CAD build for the part. Positions are in the model's coordinates, mm. A direction names the side the tool comes from. Round coordinates to 2 decimals unless told otherwise and drop trailing zeros. Loops run counter-clockwise (first coordinate to the right, second up) from the corner with the lowest first, then second, coordinate; pieces in that order, holes last. Notation, with made-up numbers: M 6,52 L 48,52 A18 cw 48,58 Z; hole C 22,-5 d1. An arc over 180 degrees is marked long. Put each result on its own line as item: value. Start each with the question number.
from build123d import *

# Parameters (mm, degrees)
PAD_DEPTH       = 5
FILLET_R        = 1
FILLET001_R     = 1
FILLET002_R     = 1
SKETCH001_R     = 1.75
PAD001_DEPTH    = 2
SKETCH002_W     = 61.2
SKETCH002_H     = 76.2
PAD002_DEPTH    = 2
PAD003_DEPTH    = 55
SKETCH004_W     = 35
SKETCH004_H     = 25
SKETCH004_W_2   = 14.2
SKETCH004_H_2   = 19
SKETCH004_W_3   = 51.2
SKETCH004_H_3   = 20
POCKET_DEPTH    = 2
SKETCH005_W     = 14.2
SKETCH005_H     = 19
SKETCH005_W_2   = 51.2
SKETCH005_H_2   = 20
POCKET001_DEPTH = 2
SKETCH006_W     = 66.2
SKETCH006_H     = 22
SKETCH006_H_2   = 17
POCKET002_DEPTH = 2
SKETCH007_W     = 24.2
SKETCH007_H     = 10
SKETCH007_W_2   = 31.5
SKETCH007_H_2   = 12
SKETCH007_R     = 1.25
PAD004_DEPTH    = 2
SKETCH008_W     = 31.5
SKETCH008_H     = 2
PAD005_DEPTH    = 3
PAD006_DEPTH    = 2
SKETCH010_W     = 5
SKETCH010_H     = 3
PAD007_DEPTH    = 2
SKETCH011_W     = 6
SKETCH011_H     = 6
SKETCH011_R     = 1.25
PAD008_DEPTH    = 6
SKETCH012_W     = 2
SKETCH012_H     = 10
PAD009_DEPTH    = 25


with BuildPart() as part:
    # Sketch → Pad (new body)
    with BuildSketch(Plane.XY):
        Polygon((28.537386, 0), (-14.268693, 24.714102), (-14.268693, -24.714102), align=None)
        Polygon((24.537386, 0), (-12.268693, 21.25), (-12.268693, -21.25), align=None, mode=Mode.SUBTRACT)
    extrude(amount=PAD_DEPTH)

    # Fillet
    fillet_edges = [part.edges().sort_by_distance(p)[0] for p in [
        (-14.268693, -24.714102, 2.5),
    ]]
    fillet(fillet_edges, radius=FILLET_R)

    # Fillet001
    fillet001_edges = [part.edges().sort_by_distance(p)[0] for p in [
        (28.537386, 0, 2.5),
    ]]
    fillet(fillet001_edges, radius=FILLET001_R)

    # Fillet002
    fillet002_edges = [part.edges().sort_by_distance(p)[0] for p in [
        (-14.268693, 24.714102, 2.5),
    ]]
    fillet(fillet002_edges, radius=FILLET002_R)

    # Sketch001 (on Face1 of Fillet002) → Pad001 (join)
    with BuildSketch(Plane(origin=(0, 0, 0), x_dir=(1, 0, 0), z_dir=(0, 0, -1))):
        Polygon((24.537386, 0), (-12.268693, 21.25), (-12.268693, -21.25), align=None)
        with Locations((4.134347, 7.160898)):
            Circle(SKETCH001_R, mode=Mode.SUBTRACT)
        with Locations((4.134347, -7.160898)):
            Circle(SKETCH001_R, mode=Mode.SUBTRACT)
        with Locations((-8.268693, 0)):
            Circle(SKETCH001_R, mode=Mode.SUBTRACT)
        Polygon((8.537386, 0), (-4.268693, 7.393594), (-4.268693, -7.393594), align=None, mode=Mode.SUBTRACT)
    extrude(amount=-PAD001_DEPTH)

    # Sketch002 (on Face9 of Pad001) → Pad002 (join)
    with BuildSketch(Plane.XY.offset(5)):
        with Locations((-1.062614, -0.09)):
            Rectangle(SKETCH002_W, SKETCH002_H)
        Polygon((-12.268693, 21.25), (-12.268693, -21.25), (24.537386, 0), align=None, mode=Mode.SUBTRACT)
    extrude(amount=PAD002_DEPTH)

    # Sketch003 (on Face21 of Pad002) → Pad003 (join)
    with BuildSketch(Plane.XY.offset(7)):
        Polygon((-31.662614, 38.01), (29.537386, 38.01), (29.537386, -38.19), (-31.662614, -38.19), (-31.662614, -36.19), (27.537386, -36.19), (27.537386, 36.01), (-31.662614, 36.01), align=None)
    extrude(amount=PAD003_DEPTH)

    # Sketch004 (on Face26 of Pad003) → Pocket (cut)
    with BuildSketch(Plane.XZ.offset(38.19)):
        with Locations((10.037386, 19.5)):
            Rectangle(SKETCH004_W, SKETCH004_H)
        with Locations((-19.562614, 19.5)):
            Rectangle(SKETCH004_W_2, SKETCH004_H_2)
        with Locations((-1.062614, 47)):
            Rectangle(SKETCH004_W_3, SKETCH004_H_3)
    extrude(amount=-POCKET_DEPTH, mode=Mode.SUBTRACT)

    # Sketch005 (on Face21 of Pocket) → Pocket001 (cut)
    with BuildSketch(Plane(origin=(0, 38.01, 0), x_dir=(-1, 0, 0), z_dir=(0, 1, 0))):
        Polygon((-24.537386, 32), (-12.537386, 32), (-12.537386, 34), (7.462614, 34), (7.462614, 32), (7.462614, 10), (-24.537386, 10), align=None)
        with Locations((19.562614, 19.5)):
            Rectangle(SKETCH005_W, SKETCH005_H)
        with Locations((1.062614, 47)):
            Rectangle(SKETCH005_W_2, SKETCH005_H_2)
    extrude(amount=-POCKET001_DEPTH, mode=Mode.SUBTRACT)

    # Sketch006 (on Face25 of Pocket001) → Pocket002 (cut)
    with BuildSketch(Plane.YZ.offset(29.537386)):
        with Locations((-0.09, 21)):
            Rectangle(SKETCH006_W, SKETCH006_H)
        with Locations((-0.09, 48.5)):
            Rectangle(SKETCH006_W, SKETCH006_H_2)
    extrude(amount=-POCKET002_DEPTH, mode=Mode.SUBTRACT)

    # Sketch007 (on Face62 of Pocket002) → Pad004 (join)
    with BuildSketch(Plane(origin=(0, 0, 32), x_dir=(1, 0, 0), z_dir=(0, 0, -1))):
        Polygon((-31.662614, 36.19), (27.537386, 36.19), (27.537386, -36.01), (12.537386, -36.01), (12.537386, -26.01), (17.537386, -26.01), (17.537386, 26.19), (-31.662614, 26.19), align=None)
        with Locations((-19.562614, -31.01)):
            Rectangle(SKETCH007_W, SKETCH007_H)
        with Locations((45.287386, -32.01)):
            Rectangle(SKETCH007_W_2, SKETCH007_H_2)
        with Locations((58.037386, -32.91)):
            Circle(SKETCH007_R, mode=Mode.SUBTRACT)
        with Locations((32.037386, -32.91)):
            Circle(SKETCH007_R, mode=Mode.SUBTRACT)
        with Locations((45.287386, 32.19)):
            Rectangle(SKETCH007_W_2, SKETCH007_H_2)
        with Locations((32.037386, 33.09)):
            Circle(SKETCH007_R, mode=Mode.SUBTRACT)
        with Locations((58.037386, 33.09)):
            Circle(SKETCH007_R, mode=Mode.SUBTRACT)
    extrude(amount=-PAD004_DEPTH)

    # Sketch008 (on Face78 of Pad004) → Pad005 (join, symmetric)
    with BuildSketch(Plane.XY.offset(34)):
        with Locations((45.287386, 37.01)):
            Rectangle(SKETCH008_W, SKETCH008_H)
        with Locations((45.287386, -37.19)):
            Rectangle(SKETCH008_W, SKETCH008_H)
    extrude(amount=PAD005_DEPTH, both=True)

    # Sketch009 (on Face31 of Pad005) → Pad006 (join)
    with BuildSketch(Plane.XY.offset(62)):
        Polygon((-31.662614, 36.01), (27.537386, 36.01), (27.537386, -36.19), (-31.662614, -36.19), (-31.662614, -34.19), (-31.662614, -31.19), (-27.662614, -31.19), (-27.662614, -34.19), (25.537386, -34.19), (25.537386, 34.01), (-27.662614, 34.01), (-27.662614, 31.01), (-31.662614, 31.01), (-31.662614, 34.01), align=None)
    extrude(amount=-PAD006_DEPTH)

    # Sketch010 (on Face24 of Pad006) → Pad007 (join)
    with BuildSketch(Plane(origin=(-31.662614, 0, 0), x_dir=(0, -1, 0), z_dir=(-1, 0, 0))):
        with Locations((-33.51, 58.5)):
            Rectangle(SKETCH010_W, SKETCH010_H)
        with Locations((33.69, 58.5)):
            Rectangle(SKETCH010_W, SKETCH010_H)
    extrude(amount=-PAD007_DEPTH)

    # Sketch011 (on Face17 of Pad007) → Pad008 (join)
    with BuildSketch(Plane(origin=(-31.662614, 0, 0), x_dir=(0, -1, 0), z_dir=(-1, 0, 0))):
        with Locations((31.19, 2)):
            Rectangle(SKETCH011_W, SKETCH011_H)
        with Locations((31.19, 2)):
            Circle(SKETCH011_R, mode=Mode.SUBTRACT)
        with Locations((-8.81, 2)):
            Rectangle(SKETCH011_W, SKETCH011_H)
        with Locations((-8.81, 2)):
            Circle(SKETCH011_R, mode=Mode.SUBTRACT)
    extrude(amount=-PAD008_DEPTH)

    # Sketch012 (on Face119 of Pad008) → Pad009 (join)
    with BuildSketch(Plane(origin=(0, 0, 32), x_dir=(1, 0, 0), z_dir=(0, 0, -1))):
        with Locations((-8.462614, 31.19)):
            Rectangle(SKETCH012_W, SKETCH012_H)
        with Locations((-8.462614, -31.01)):
            Rectangle(SKETCH012_W, SKETCH012_H)
    extrude(amount=PAD009_DEPTH)


solid = part.part
(1) Cut at A-A on z = 12. Count the separate pieces of the cut face and the enclosed holes in it, and give its area (3 significant figures).
(2) Drill centre lines: line 1 along Z through (x, y) = (-27.3, -31.19); line 2 along X through (y, z) = (-33.09, 33.1); line 3 along Z through (x, y) = (22, 23). Where is each one in solid material? Low to high.
(3) Flat gauge pins, fed straight in: pin 1 Ø10 at (y, z) = (-1.5, 41) entering from -X; pin 2 Ø5 at (x, y) = (48.5, 32) entering from +Z; pin 3 Ø1.5 at (x, y) = (7, 9) entering from -Z. Where does each tip first touch, or does it go through?
(4) Tool access for faces 4 (the flat face through (-9, 26.01, 27)), 5 (the flat face through (45, -36.19, 36)), 6 (the flat face through (2.224, -3.645, 0.986)), 7 (the flat face through (-29, -28.19, 2)): list every direction of +Z, -Z, +X, -X, +Y, -Y with a clear straight run to the whole face (end or side of a thin tool).
(5) Cut at D-D on y = 17.5. List the corners of the cut face in (x, z), and give its area (3 significant figures).
(6) Mould opens along Z. For faces 1 (the flat face through (27.537, -7, 9)), 2 (the flat face through (-29, 9, -1)), 3 (the flat face through (-25.663, -31.1, 3.4)) say: +Z half, -Z half, draft (parallel to the pull), parting line (faces both ways), or undercut.
Taken from the geometry:
1. separate pieces: 6
1. enclosed holes: 0
1. area: 106 mm2
2. line 1: -1 to 0.75, 3.25 to 7, 32 to 34
2. line 2: -31.66 to 30.79, 33.29 to 56.79, 59.29 to 61.04
2. line 3: 5 to 7, 32 to 34
3. pin 1: x = 27.54
3. pin 2: z = 34
3. pin 3: z = 0
4. face 4: +Z, -X
4. face 5: +Z, +X
4. face 6: +Z, -Z
4. face 7: -Z, +X, -X
5. outline: M -31.66,5 L -14.27,5 L -14.27,0 L -1.77,0 L -1.77,5 L 29.54,5 L 29.54,10 L 27.54,10 L 27.54,7 L -5.77,7 L -5.77,2 L -12.27,2 L -12.27,7 L -31.66,7 Z; M 17.54,32 L 29.54,32 L 29.54,40 L 27.54,40 L 27.54,34 L 17.54,34 Z; M 25.54,60 L 27.54,60 L 27.54,57 L 29.54,57 L 29.54,62 L 25.54,62 Z
5. area: 208 mm2
6. face 1: undercut
6. face 2: -Z half
6. face 3: draft
